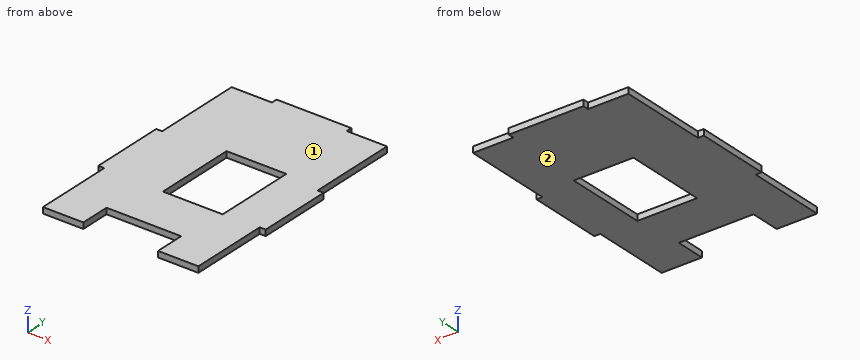
from build123d import *

# Parameters (mm, degrees)
SKETCH_2_W          = 112
SKETCH_2_H          = 172
EXTRUDE_1_DEPTH     = 4
SKETCH_3_W          = 27
SKETCH_3_H          = 4
SKETCH_3_W_2        = 4
SKETCH_3_H_2        = 58
CUT_EXTRUDE_2_DEPTH = 4
SKETCH_5_W          = 104
SKETCH_5_H          = 5
CUT_EXTRUDE_4_DEPTH = 4
SKETCH_6_W          = 40
SKETCH_6_H          = 55
CUT_EXTRUDE_5_DEPTH = 4
SKETCH_8_W          = 50
SKETCH_8_H          = 20
CUT_EXTRUDE_6_DEPTH = 4


with BuildPart() as part:
    # 스케치2 → 보스-돌출1 (new body)
    with BuildSketch(Plane.XY):
        with Locations((56, 1)):
            Rectangle(SKETCH_2_W, SKETCH_2_H)
    extrude(amount=-EXTRUDE_1_DEPTH)

    # 스케치3 → 컷-돌출2 (cut)
    with BuildSketch(Plane.XY):
        with Locations((94.5, 85)):
            Rectangle(SKETCH_3_W, SKETCH_3_H)
        Polygon((112, 23), (112, 87), (108, 87), (108, 83), (108, 23), align=None)
        with Locations((17.5, 85)):
            Rectangle(SKETCH_3_W, SKETCH_3_H)
        Polygon((4, 83), (4, 87), (0, 87), (0, 23), (4, 23), align=None)
        with Locations((2, -56)):
            Rectangle(SKETCH_3_W_2, SKETCH_3_H_2)
        with Locations((110, -56)):
            Rectangle(SKETCH_3_W_2, SKETCH_3_H_2)
    extrude(amount=-CUT_EXTRUDE_2_DEPTH, mode=Mode.SUBTRACT)

    # 스케치5 → 컷-돌출4 (cut)
    with BuildSketch(Plane.XY):
        with Locations((56, -82.5)):
            Rectangle(SKETCH_5_W, SKETCH_5_H)
    extrude(amount=-CUT_EXTRUDE_4_DEPTH, mode=Mode.SUBTRACT)

    # 스케치6 → 컷-돌출5 (cut)
    with BuildSketch(Plane.XY):
        with Locations((64, -0.5)):
            Rectangle(SKETCH_6_W, SKETCH_6_H)
    extrude(amount=-CUT_EXTRUDE_5_DEPTH, mode=Mode.SUBTRACT)

    # 스케치8 → 컷-돌출6 (cut)
    with BuildSketch(Plane.XY):
        with Locations((56, -70)):
            Rectangle(SKETCH_8_W, SKETCH_8_H)
    extrude(amount=-CUT_EXTRUDE_6_DEPTH, mode=Mode.SUBTRACT)


solid = part.part
Input: part model. Units: mm. Frame: model coordinates. Face numbers are marked on the shaded views. Round coordinates to 2 decimals unless told otherwise and drop trailing zeros. Loops run counter-clockwise (first coordinate to the right, second up) from the corner with the lowest first, then second, coordinate; pieces in that order, holes last. Notation, with made-up numbers: (60, 88.25) -> (119, 88.25) arc R15 ccw to (119, 100.25) -> close; hole circle Ø1 at (46.5, 59.5). An arc over 180 degrees is marked (long way). Answer as a JSON object with one key per item and string values. Group by question number.
1) Section query B-B on x = 61.5. Output: boundary loops of the cut face in (y, z), plus the area to 3 significant figures.
2) Pin query (flat end, axial travel): pin 1 (2 mm diameter, centred on y = -43, z = -2, fed in from +X); pin 2 (1.2 mm diameter, centred on y = -52.5, z = -2.5, fed in from -X); pin 3 (2 mm diameter, centred on x = 95.5, z = -3, fed in from +Y). Return the tip coordinate at first contact, or that it passes through.
3) Draft query along Z for the marked faces 1 and 2. Return one class per face: +Z half, -Z half, draft (parallel to the pull), parting line (faces both ways), or undercut.
4) Section query D-D on x = 17.5. Output: boundary loops of the cut face in (y, z), plus the area to 3 significant figures.
5) Section query C-C on z = -3.2. Output: boundary loops of the cut face in (x, y), plus the area to 3 significant figures.
6) Section query A-A on y = -24.5. Output: boundary loops of the cut face in (x, z).
7) Ray query, L1, parallel to Y at x = 57, z = -3.2; L2, parallel to X at y = 11.5, z = -2.9; L3, parallel to X at y = -64, z = -3.2. Return the intervals inside material, ascending.
Reply:
{
 "1": {"outline": "(-60, -4) -> (-28, -4) -> (-28, 0) -> (-60, 0) -> close; (27, -4) -> (87, -4) -> (87, 0) -> (27, 0) -> close", "area": "368 mm2"},
 "2": {"pin 1": "stops at x = 108", "pin 2": "stops at x = 4", "pin 3": "stops at y = 83"},
 "3": {"face 1": "+Z half", "face 2": "-Z half"},
 "4": {"outline": "(-80, -4) -> (83, -4) -> (83, 0) -> (-80, 0) -> close", "area": "652 mm2"},
 "5": {"outline": "(0, -27) -> (4, -27) -> (4, -80) -> (31, -80) -> (31, -60) -> (81, -60) -> (81, -80) -> (108, -80) -> (108, -27) -> (112, -27) -> (112, 23) -> (108, 23) -> (108, 83) -> (81, 83) -> (81, 87) -> (31, 87) -> (31, 83) -> (4, 83) -> (4, 23) -> (0, 23) -> close; hole (44, -28) -> (84, -28) -> (84, 27) -> (44, 27) -> close", "area": "14,400 mm2"},
 "6": {"outline": "(0, -4) -> (44, -4) -> (44, 0) -> (0, 0) -> close; (84, -4) -> (112, -4) -> (112, 0) -> (84, 0) -> close"},
 "7": {"L1": "y = -60 to -28, 27 to 87", "L2": "x = 0 to 44, 84 to 112", "L3": "x = 4 to 31, 81 to 108"}
}
